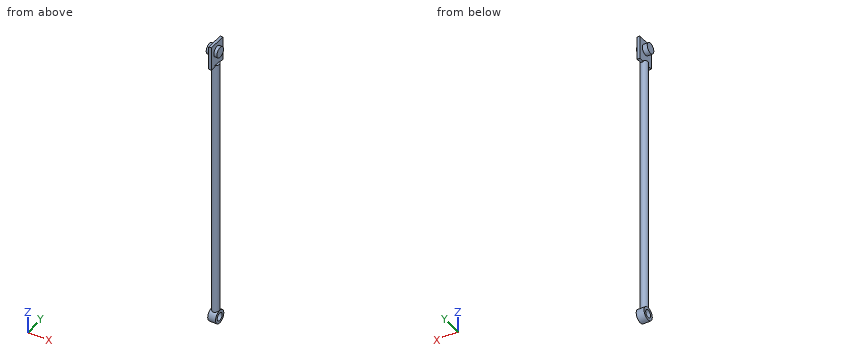
from build123d import *

# Parameters (mm, degrees)
SKETCH1_R                = 1.4
BOSS_EXTRUDE1_DEPTH      = 100
SKETCH2_W                = 3
SKETCH2_H                = 1
SKETCH3_W                = 1
SKETCH3_H                = 7
BOSS_EXTRUDE2_DEPTH      = 9
BOSS_EXTRUDE3_DEPTH      = 1.7
BOSS_EXTRUDE3_DEPTH_BACK = 2.4
SKETCH4_R                = 2


with BuildPart() as part:
    # Sketch1 → Boss-Extrude1 (new body)
    with BuildSketch(Plane.XY):
        Circle(SKETCH1_R)
    extrude(amount=BOSS_EXTRUDE1_DEPTH)

    # Sketch2 → Revolve1 (revolve)
    with BuildSketch(Plane(origin=(0, 0, 0), x_dir=(1, 0, 0), z_dir=(0, 1, 0))):
        Rectangle(SKETCH2_W, SKETCH2_H)
    revolve(axis=Axis((-2.442552493, 0, -2), (1, 0, 0)))

    # Sketch3 → Boss-Extrude2 (add)
    with BuildSketch(Plane.XY.offset(99.5)):
        Rectangle(SKETCH3_W, SKETCH3_H)
    extrude(amount=BOSS_EXTRUDE2_DEPTH)

    # Sketch4 → Boss-Extrude3 (add, two sides: drawn at the far end of the back side and taken through both)
    with BuildSketch(Plane(origin=(0, 0, 0), x_dir=(0, 0, -1), z_dir=(1, 0, 0)).offset(-BOSS_EXTRUDE3_DEPTH_BACK)):
        with Locations((-105, 0)):
            Circle(SKETCH4_R)
    extrude(amount=BOSS_EXTRUDE3_DEPTH + BOSS_EXTRUDE3_DEPTH_BACK)


solid = part.part
Could you check a few things on this model? Use its own coordinates, in mm. Give positions to 0.01 mm unless a question says otherwise; leave off trailing zeros. Order: outer loops, then holes, each group sorted by start corner. A loop starts at its lowest first (then second) coordinate and runs counter-clockwise, first axis right, second up. Notation, with made-up numbers: (72.25, -32) - (78.25, -32) arc R32 cw to (78.25, -2) - close; hole circle Ø7 at (-1.75, 71). An arc over 180 degrees is marked (long way). One line per question, with ' | ' between items. Start each with the question number.
Item 1: I'm going to push flat-ended pins straight in: pin 1 Ø4 at (y, z) = (0, 67) entering from +X; pin 2 Ø4 at (y, z) = (-0.5, -2.5) entering from -X; pin 3 Ø1.5 at (y, z) = (0.5, -2) entering from +X; pin 4 Ø0.8 at (x, y) = (0, 2.5) entering from -Z. Where does each tip first touch, or does it pass through?
Item 2: I want a section at A-A on z = -2. Write out the boundary of the cut face in (x, y), then the cut area to 3 significant figures.
Item 3: I need wall thicknesses on probe 1 along Z at (x, y) = (-0.75, 0); probe 2 along Z at (x, y) = (-0.15, 0); probe 3 along Y at (x, z) = (-0.4, -2). Which ranges of each line are inside material? Lowest first, please. Write a range as [from, to].
Item 4: I want a section at C-C on z = 85. Write out the boundary of the cut face in (x, y).
Item 5: I want a section at B-B on z = 105. Write out the boundary of the cut face in (x, y).
Verdict:
1) pin 1: x = 1.4 | pin 2: x = -1.5 | pin 3: through | pin 4: z = -3.36
2) outline: (-1.5, -2.5) - (1.5, -2.5) - (1.5, -1.5) - (-1.5, -1.5) - close; (-1.5, 1.5) - (1.5, 1.5) - (1.5, 2.5) - (-1.5, 2.5) - close | area: 6.00 mm^2
3) probe 1: [-4.5, -3.5], [-0.5, 100], [103, 107] | probe 2: [-4.5, -3.5], [-0.5, 108.5] | probe 3: [-2.5, -1.5], [1.5, 2.5]
4) outline: circle Ø2.8 at (0, 0)
5) outline: (-2.4, -2) - (-0.5, -2) - (-0.5, -3.5) - (0.5, -3.5) - (0.5, -2) - (1.7, -2) - (1.7, 2) - (0.5, 2) - (0.5, 3.5) - (-0.5, 3.5) - (-0.5, 2) - (-2.4, 2) - close
